Source: CAD feature listing. Evaluate the final solid. Frame: model axes, mm. Face numbers are marked on the shaded views. A direction names the side the tool comes from. Coordinates: 2 decimals unless noted, no trailing zeros. Order: outer loops, then holes, each group sorted by start corner. A loop starts at its lowest first (then second) coordinate and runs counter-clockwise, first axis right, second up. Notation, with made-up numbers: (6.5, -32.5) -> (60.5, -32.5) arc R27 ccw to (60.5, 5.5) -> close; hole circle Ø11 at (-14, -32). An arc over 180 degrees is marked (long way). Write item = value, one per line. Start each with the question number.
Item 1: Section query B-B (z = -31.5). Output: boundary loops of the cut face in (x, y).
Item 2: Section query A-A (x = 39). Output: boundary loops of the cut face in (y, z), then the cut area to 3 significant figures.
Item 3: Section query C-C (z = -11.5). Output: boundary loops of the cut face in (x, y).
Item 4: Set-up query: the marked faces 1, 2 and 3. Return all of +Z, -Z, +X, -X, +Y, -Y with unobstructed straight access to the full face (end or side cutting, diameter ignored); none if empty.
Item 5: Section query D-D (x = 7.5). Output: boundary loops of the cut face in (y, z).
Item 6: Contact query for flat-ended pins moving along their axis: pin 1 (3.5 mm diameter, centred on x = 39, z = -31.5, fed in from +Y); pin 2 (3 mm diameter, centred on x = 9, y = 9, fed in from -Z); pin 3 (4 mm diameter, centred on y = 9.5, z = -5.5, fed in from -X). Output: stop coordinate, or through.
Item 7: Ray query, line 1 along X through (y, z) = (2.95, -31.5); line 2 along Z through (x, y) = (4.5, 7.75); line 3 along Y through (x, z) = (-38, -14). Return the intervals inside material, ascending. Write a range as [from, to].
```python
from build123d import *

# Parameters (mm, degrees)
SKETCH1_W           = 84
SKETCH1_H           = 69
BOSS_EXTRUDE1_DEPTH = 6
SKETCH2_W           = 72
SKETCH2_H           = 25
BOSS_EXTRUDE2_DEPTH = 7
SKETCH3_R           = 1.6
CUT_EXTRUDE1_DEPTH  = 55.801916025
SKETCH4_R           = 1.6
CUT_EXTRUDE2_DEPTH  = 55.801916025
SKETCH5_R           = 1.6
CUT_EXTRUDE3_DEPTH  = 55.801916025
SKETCH6_R           = 1.6
CUT_EXTRUDE4_DEPTH  = 55.801916025


with BuildPart() as part:
    # Sketch1 → Boss-Extrude1 (new body)
    with BuildSketch(Plane(origin=(0, 0, 0), x_dir=(1, 0, 0), z_dir=(0, 1, 0))):
        Rectangle(SKETCH1_W, SKETCH1_H)
    extrude(amount=BOSS_EXTRUDE1_DEPTH)

    # Sketch2 → Boss-Extrude2 (add)
    with BuildSketch(Plane(origin=(0, 6, 0), x_dir=(1, 0, 0), z_dir=(0, 1, 0))):
        with Locations((0, 14)):
            Rectangle(SKETCH2_W, SKETCH2_H)
    extrude(amount=BOSS_EXTRUDE2_DEPTH)

    # Sketch3 → Cut-Extrude1 (cut, through all)
    with BuildSketch(Plane(origin=(0, 6, 0), x_dir=(1, 0, 0), z_dir=(0, 1, 0))):
        with Locations(Location((-39, 31.5, 0), (0, 0, 270))):
            Circle(SKETCH3_R)
    extrude(amount=-CUT_EXTRUDE1_DEPTH, mode=Mode.SUBTRACT)

    # Sketch4 → Cut-Extrude2 (cut, through all)
    with BuildSketch(Plane(origin=(0, 6, 0), x_dir=(1, 0, 0), z_dir=(0, 1, 0))):
        with Locations(Location((39, 31.5, 0), (0, 0, 270))):
            Circle(SKETCH4_R)
    extrude(amount=-CUT_EXTRUDE2_DEPTH, mode=Mode.SUBTRACT)

    # Sketch5 → Cut-Extrude3 (cut, through all)
    with BuildSketch(Plane(origin=(0, 6, 0), x_dir=(1, 0, 0), z_dir=(0, 1, 0))):
        with Locations(Location((-39, 1.5, 0), (0, 0, 270))):
            Circle(SKETCH5_R)
    extrude(amount=-CUT_EXTRUDE3_DEPTH, mode=Mode.SUBTRACT)

    # Sketch6 → Cut-Extrude4 (cut, through all)
    with BuildSketch(Plane(origin=(0, 6, 0), x_dir=(1, 0, 0), z_dir=(0, 1, 0))):
        with Locations(Location((39, 1.5, 0), (0, 0, 270))):
            Circle(SKETCH6_R)
    extrude(amount=-CUT_EXTRUDE4_DEPTH, mode=Mode.SUBTRACT)


solid = part.part
```
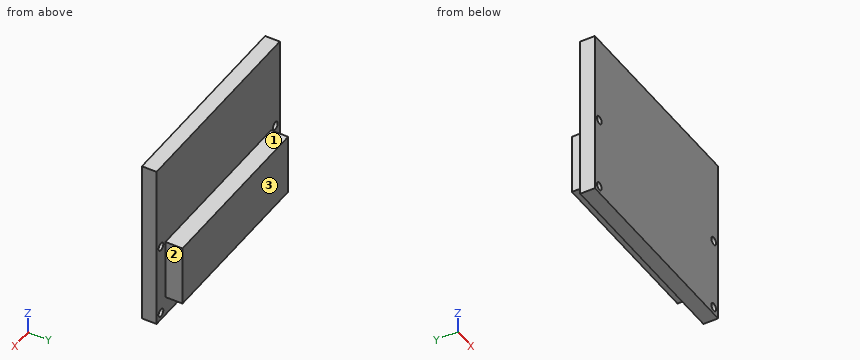
Computed:
q1.outline = (-42, 0) -> (-40.6, 0) -> (-40.6, 6) -> (-42, 6) -> close; (-37.4, 0) -> (37.4, 0) -> (37.4, 6) -> (-37.4, 6) -> close; (40.6, 0) -> (42, 0) -> (42, 6) -> (40.6, 6) -> close
q2.outline = (0, -34.5) -> (6, -34.5) -> (6, -33.1) -> (0, -33.1) -> close; (0, -29.9) -> (6, -29.9) -> (6, -3.1) -> (0, -3.1) -> close; (0, 0.1) -> (6, 0.1) -> (6, 34.5) -> (0, 34.5) -> close
q2.area = 376 mm^2
q3.outline = (-42, 0) -> (42, 0) -> (42, 6) -> (36, 6) -> (36, 13) -> (-36, 13) -> (-36, 6) -> (-42, 6) -> close
q4.face_1 = +Z, +X, -X, +Y
q4.face_2 = +Z, -Z, +X, +Y
q4.face_3 = +Z, -Z, +X, -X, +Y
q5.outline = (0, -34.5) -> (6, -34.5) -> (6, -26.5) -> (13, -26.5) -> (13, -1.5) -> (6, -1.5) -> (6, 34.5) -> (0, 34.5) -> close
q6.pin_1 = 6
q6.pin_2 = -26.5
q6.pin_3 = -36
q7.line_1 = [-42, -40.6], [-37.4, 37.4], [40.6, 42]
q7.line_2 = [-26.5, -1.5]
q7.line_3 = [0, 6]
